Geometry check sheet. Reference: the model listing, model coordinates, mm. Round coordinates to 2 decimals unless told otherwise and drop trailing zeros. Order: outer loops, then holes, each group sorted by start corner. A loop starts at its lowest first (then second) coordinate and runs counter-clockwise, first axis right, second up. Notation, with made-up numbers: (35.25, 76.25) - (89.25, 76.25) arc R15 ccw to (89.25, 85.25) - close; hole circle Ø1 at (-5.75, 11.5). An arc over 180 degrees is marked (long way). Return JSON: item names as keys, results as strings. Group by question number.
Q1. Sectioned sample at C-C, the plane z = -323. Record the cut outline in (x, y).
Q2. Sectioned sample at B-B, the plane x = -500. Record the cut outline in (y, z).
Q3. Sectioned sample at A-A, the plane y = -2.25. Record the cut outline in (x, z).
Q4. Gauge pin test, flat ends, axial feed: pin 1 Ø4 at (y, z) = (-11, 67) entering from -X; pin 2 Ø6.5 at (x, y) = (-604, -6.5) entering from +Z. Record the tip position at first contact, or that the pin passes through.
Q5. Material ranges on line 1 along Z through (x, y) = (-453, -7.5); line 2 along Z through (x, y) = (-361.5, -5.5); line 3 along X through (y, z) = (-8.75, 56.5), recorded low to high.
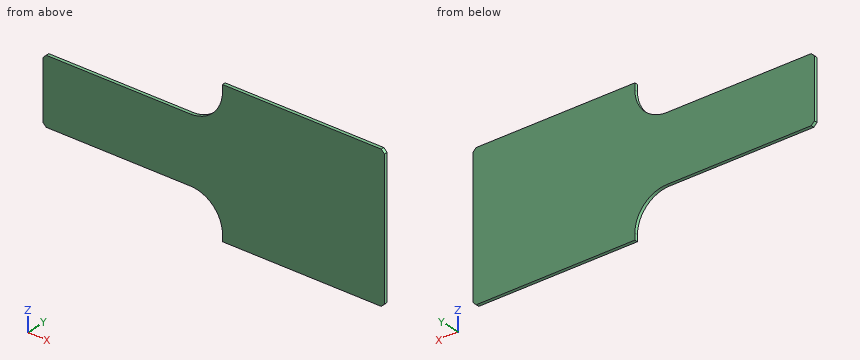
```python
from build123d import *

# Parameters (mm, degrees)
F1_DEPTH = 12.7
F2_SIZE  = 12.7


with BuildPart() as f1:
    # F0 (on Front) → F1 (new body)
    with BuildSketch(Plane.XZ):
        with BuildLine():
            Line((399.451222, -412.90055), (399.451222, 149.86185))
            Line((399.451222, 149.86185), (-241.898778, 149.86185))
            Line((-241.898778, 149.86185), (-241.898778, 124.46185))
            ThreePointArc((-241.898778, 124.46185), (-279.096217, 34.659289), (-368.898778, -2.53815))
            Line((-368.898778, -2.53815), (-953.098778, -2.53815))
            Line((-953.098778, -2.53815), (-953.098778, -260.50055))
            Line((-953.098778, -260.50055), (-368.898778, -260.50055))
            ThreePointArc((-368.898778, -260.50055), (-279.096217, -297.697989), (-241.898778, -387.50055))
            Line((-241.898778, -387.50055), (-241.898778, -412.90055))
            Line((-241.898778, -412.90055), (399.451222, -412.90055))
        make_face()
    extrude(amount=F1_DEPTH)

    # F2
    f2_edges = [f1.edges().sort_by_distance(p)[0] for p in [
        (-953.098778, -6.35, -2.53815),
        (-953.098778, -6.35, -260.50055),
        (399.451222, -6.35, -412.90055),
        (399.451222, -6.35, 149.86185),
    ]]
    chamfer(f2_edges, length=F2_SIZE)


solid = f1.part
```
Reply:
{
 "1": {"outline": "(-259.5, -12.7) - (399.45, -12.7) - (399.45, 0) - (-259.5, 0) - close"},
 "2": {"outline": "(-12.7, -260.5) - (0, -260.5) - (0, -2.54) - (-12.7, -2.54) - close"},
 "3": {"outline": "(-953.1, -247.8) - (-940.4, -260.5) - (-368.9, -260.5) arc R127 cw to (-241.9, -387.5) - (-241.9, -412.9) - (386.75, -412.9) - (399.45, -400.2) - (399.45, 137.16) - (386.75, 149.86) - (-241.9, 149.86) - (-241.9, 124.46) arc R127 cw to (-368.9, -2.54) - (-940.4, -2.54) - (-953.1, -15.24) - close"},
 "4": {"pin 1": "x = -256.68", "pin 2": "z = -2.54"},
 "5": {"line 1": "-260.5 to -2.54", "line 2": "-260.72 to -2.32", "line 3": "-261.61 to 399.45"}
}
